Geometry check sheet. Reference: the model listing, model coordinates, mm. A direction names the side the tool comes from. Give positions to 0.01 mm unless a question says otherwise; leave off trailing zeros. Write each loop counter-clockwise with the first axis right and the second up, starting at its lowest first coordinate (ties: lowest second). Pieces come first, ordered by that corner, then holes.
(1) Cross-section at C-C (x = 3.5). Record the boundary of the cut face in (y, z), and give its area (3 significant figures).
(2) Cross-section at A-A (z = 7.95). Record the boundary of the cut face in (x, y).
(3) Cross-section at D-D (y = -1). Record the boundary of the cut face in (x, z).
(4) Cross-section at B-B (x = 15). Record the boundary of the cut face in (y, z).
(5) Thickness scan on line 1 along Y through (x, z) = (2.95, 7.95); line 2 along Z through (x, y) = (6.5, -6); line 3 along Z through (x, y) = (0.7, 7). Record the ranges inside material, lowest first.
(6) Mould release check, pull along Y, two halves, no side actions. Record for faces 6 (the cylindrical face through (1.972, 10.536, -8.275)), 7 (the flat face through (12, 0, -11.15)), 8 (the cylindrical face through (0.99, 11.77, -1.5)), 9 (the flat face through (6, 15.2, 0)): +Y half, -Y half, draft (parallel to the pull), parting line (faces both ways), or undercut.
(7) Depth check by flat-ended pin: P1, Ø16, axis at y = 7, z = 0, coming from the +X side; P2, Ø5, axis at y = 7, z = -11, coming from the -X side; P3, Ø1, axis at x = 16.5, z = 9.5, coming from the -Y side; P4, Ø1.9, axis at y = 18, z = -4, coming from the +X side. Enter the tip coordinate at first touch or a pass-through.
(8) Tool access check on faces 1 (the flat face through (10, 2, -14.95)), 2 (the flat face through (4, 0, 0)), 3 (the cylindrical face through (0.99, -2.23, -1.5)), 4 (the cylindrical face through (1.972, -13.464, -8.275)), 5 (the flat face through (13, 17, -9.95)). Record the directions out of +Z, -Z, +X, -X, +Y, -Y that give a thin tool (end or side, any length) a straight path to the whole face; none if there is none.
Autodesk Inventor part; units mm, degrees
ref_plane "YZ Plane" through (0, 0, 0) normal (1, 0, 0) x (0, 1, 0)
ref_plane "XZ Plane" through (0, 0, 0) normal (0, 1, 0) x (-1, 0, 0)
sketch "Эскиз1" plane through (0, 0, 0) normal (1, 0, 0) x (0, 1, 0)
  line L0 (-15, -10.95) -> (15, -10.95)
  line L1 (15, -10.95) -> (15, 10.95)
  line L2 (15, 10.95) -> (-15, 10.95)
  line L3 (-15, 10.95) -> (-15, -10.95)
  line L4 (-15, -10.95) -> (15, 10.95) construction
  line L5 (15, -10.95) -> (-15, 10.95) construction
  circle A0 centre (7, 0) radius 5
  circle A1 centre (-7, 0) radius 5
  point P0 (0, 0)
  dimension "d0" = 30
  dimension "d1" = 21.9
  dimension "d2" = 10
  dimension "d3" = 10
  dimension "d4" = 8
  dimension "d5" = 14
  dimension "d6" = 8
  dimension "d7" = 0
extrude "Выдавливание1" add sketch "Эскиз1" along normal blind 2
sketch "Эскиз2" plane through (2, 0, 0) normal (1, 0, 0) x (0, 0, -1)
  line L0 (10.95, 15) -> (-10.95, 15)
  line L1 (10.95, -15) -> (-10.95, -15)
  line L2 (-10.95, -15) -> (-10.95, 15)
  line L3 (-10.95, 15) -> (10.95, 15)
  line L4 (10.95, 15) -> (10.95, -15)
  line L5 (10.95, -15) -> (-10.95, 15) construction
  line L6 (-10.95, -15) -> (10.95, 15) construction
  point P0 (0, 0)
extrude "Выдавливание2" add sketch "Эскиз2" along normal blind 2
sketch "Эскиз3" plane through (0, 0, 0) normal (-1, 0, 0) x (0, 0, 1)
  circle A0 centre (-7.95, 12) radius 1.5
  line L0 (-10.95, 15) -> (10.95, 15)
  line L1 (-10.95, -15) -> (-10.95, 15)
  circle A1 centre (-7.95, -12) radius 1.5
  line L2 (10.95, -15) -> (-10.95, -15)
  circle A2 centre (7.95, 12) radius 1.5
  line L3 (10.95, 15) -> (10.95, -15)
  circle A3 centre (7.95, -12) radius 1.5
  point P0 (0, 0)
  dimension "d12" = 3
  dimension "d13" = 3
  dimension "d14" = 3
  dimension "d15" = 3
  dimension "d16" = 3
  dimension "d17" = 3
  dimension "d18" = 3
  dimension "d19" = 3
  dimension "d20" = 3
extrude "Выдавливание3" cut sketch "Эскиз3" against normal up to surface (4 mm away) contours A0 | A1 | A2 | A3
ref_plane "РабПлоскость1" through (0, 10, -4) normal (1, 0, 0) x (0, 0, -1)
sketch "Эскиз4" plane through (0, 10, -4) normal (1, 0, 0) x (0, 0, -1)
  line L0 (6.95, 5) -> (-14.95, 5)
  line L1 (-14.95, 5) -> (6.95, 5)
  line L2 (6.95, 5) -> (6.95, 9)
  line L3 (6.95, 9) -> (-14.95, 9)
  line L4 (-14.95, 9) -> (-14.95, 5)
  point P0 (-4, -10)
  dimension "d23" = 4
extrude "Выдавливание4" add sketch "Эскиз4" along normal blind 6.5
sketch "Эскиз5" plane through (4, -15, -10.95) normal (0, 0, -1) x (-1, 0, 0)
  line L0 (4, 34) -> (4, 0)
  line L1 (4, 34) -> (-16, 34)
  line L2 (-16, 34) -> (-16, 0)
  line L3 (-16, 0) -> (4, 0)
  line L4 (4, 0) -> (4, 34)
  point P0 (4, 15)
  dimension "d26" = 20
extrude "Выдавливание5" add sketch "Эскиз5" along normal blind 4
sketch "Эскиз6" plane through (0, -15, 10.95) normal (0, 0, 1) x (1, 0, 0)
  line L0 (0, 0) -> (0, 34)
  line L1 (20, 34) -> (20, 0)
  line L2 (0, 0) -> (20, 0)
  line L3 (20, 0) -> (20, 34)
  line L4 (20, 34) -> (0, 34)
  line L5 (0, 34) -> (0, 0)
  point P0 (0, 15)
  point P1 (20, 0)
  point P2 (0, 34)
extrude "Выдавливание6" add sketch "Эскиз6" along normal blind 4
sketch "Эскиз7" plane through (0, -15, 10.95) normal (0, 0, -1) x (-1, 0, 0)
  line L0 (-20, 0) -> (-20, 34)
  line L1 (-20, 0) -> (-4, 0)
  line L2 (-4, 0) -> (-4, 30)
  line L3 (-4, 30) -> (-20, 30)
  line L4 (-20, 30) -> (-20, 0)
  point P0 (0, 15)
extrude "Выдавливание7" cut sketch "Эскиз7" along normal mid plane 0.2
sketch "Эскиз8" plane through (4, -15, -10.95) normal (0, 0, 1) x (1, 0, 0)
  line L0 (16, 34) -> (16, 0)
  line L1 (0, 0) -> (0, 30)
  line L2 (16, 0) -> (0, 0)
  line L3 (0, 0) -> (0, 30)
  line L4 (0, 30) -> (16, 30)
  line L5 (16, 30) -> (16, 0)
  point P0 (-4, 15)
extrude "Выдавливание8" cut sketch "Эскиз8" against normal blind 0.2
sketch "Эскиз9" plane through (0, -15, 10.95) normal (0, 0, -1) x (-1, 0, 0)
  line L0 (-20, 30) -> (-6.5, 30)
  line L1 (-6.5, 34) -> (-20, 34)
  line L2 (-20, 34) -> (-20, 30)
  line L3 (-20, 30) -> (-6.5, 30)
  line L4 (-6.5, 30) -> (-6.5, 34)
  point P0 (0, 15)
extrude "Выдавливание9" add sketch "Эскиз9" along normal blind 1
sketch "Эскиз10" plane through (4, -15, -10.95) normal (0, 0, 1) x (1, 0, 0)
  line L0 (2.5, 30) -> (2.5, 34)
  line L1 (2.5, 30) -> (16, 30)
  line L2 (2.5, 34) -> (16, 34)
  line L3 (16, 34) -> (16, 30)
  line L4 (16, 30) -> (2.5, 30)
  line L5 (2.5, 30) -> (2.5, 34)
  point P0 (-4, 15)
extrude "Выдавливание10" add sketch "Эскиз10" along normal blind 1
sketch "Эскиз11" plane through (4, 15, 11.05) normal (0, -1, 0) x (1, 0, 0)
  line L0 (0, -22.2) -> (0, 0)
  line L1 (0, -22.2) -> (16, -22.2)
  line L2 (16, -22.2) -> (16, -21)
  line L3 (2.5, -21) -> (16, -21)
  line L4 (2.5, -1.1) -> (2.5, -21)
  line L5 (16, -1.1) -> (2.5, -1.1)
  line L6 (16, 0) -> (16, -1.1)
  line L7 (16, 0) -> (0, 0)
  point P0 (-4, -11.05)
extrude "Выдавливание11" cut sketch "Эскиз11" against normal blind 0.2
properties part number "держатель магнитов на основе"
Reply:
1. outline: (-15, -14.95) - (19, -14.95) - (19, 14.95) - (-15, 14.95) - close; hole circle Ø3 at (-12, -7.95); hole circle Ø3 at (-12, 7.95); hole circle Ø3 at (12, -7.95); hole circle Ø3 at (12, 7.95)
1. area: 988 mm2
2. outline: (0, -15) - (4, -15) - (4, -13.5) - (0, -13.5) - close; (0, -10.5) - (4, -10.5) - (4, 10.5) - (0, 10.5) - close; (0, 13.5) - (4, 13.5) - (4, 15.2) - (6.5, 15.2) - (6.5, 19) - (0, 19) - close
3. outline: (0, -14.95) - (20, -14.95) - (20, -11.15) - (4, -11.15) - (4, 11.05) - (20, 11.05) - (20, 14.95) - (0, 14.95) - close
4. outline: (-15, -14.95) - (19, -14.95) - (19, -9.95) - (15.2, -9.95) - (15.2, -11.15) - (-15, -11.15) - close; (-15, 11.05) - (15.2, 11.05) - (15.2, 9.95) - (19, 9.95) - (19, 14.95) - (-15, 14.95) - close
5. line 1: y = -15 to -13.5, -10.5 to 10.5, 13.5 to 19
5. line 2: z = -14.95 to -11.15, 11.05 to 14.95
5. line 3: z = -14.95 to -5, 5 to 14.95
6. face 6: undercut
6. face 7: draft
6. face 8: undercut
6. face 9: -Y half
7. P1: stops at x = 4
7. P2: stops at x = 0
7. P3: stops at y = 15.2
7. P4: stops at x = 6.5
8. face 1: -Z, +X, -X, +Y, -Y
8. face 2: +X, -Y
8. face 3: -X
8. face 4: +X, -X
8. face 5: +X, +Y, -Y
